For this review, take the finished solid that the model builds, in its own axes (mm). A direction names the side the tool comes from. Give positions to 0.01 mm unless a question says otherwise; leave off trailing zeros. Order: outer loops, then holes, each group sorted by start corner. A loop starts at its lowest first (then second) coordinate and runs counter-clockwise, first axis right, second up. Notation, with made-up numbers: (-34, 10.5) -> (-18, 10.5) arc R34 ccw to (-18, 46.5) -> close; hole circle Ø6 at (41, 40.25). An arc over 180 degrees is marked (long way). One line per item, written item: value. Start each with the question number.
from build123d import *

# Parameters (mm, degrees)
SKETCH2_W           = 25
SKETCH2_H           = 40
BOSS_EXTRUDE3_DEPTH = 60
SKETCH13_W          = 21
SKETCH13_H          = 42
CUT_EXTRUDE5_DEPTH  = 37
SKETCH15_W          = 25
SKETCH15_H          = 7.915590507
CUT_EXTRUDE7_DEPTH  = 7.2
SKETCH16_R          = 1.5
CUT_EXTRUDE8_DEPTH  = 8
SKETCH17_W          = 25
SKETCH17_H          = 36
CUT_EXTRUDE9_DEPTH  = 7.2
SKETCH19_W          = 20
SKETCH19_H          = 29
CUT_EXTRUDE10_DEPTH = 4
SKETCH23_R          = 2
CUT_EXTRUDE12_DEPTH = 10
SKETCH24_W          = 5.82179869
SKETCH24_H          = 4.560057011
SKETCH24_W_2        = 6.048044386
CUT_EXTRUDE14_DEPTH = 1
SKETCH25_W          = 3.2
SKETCH25_H          = 3.755693487
CUT_EXTRUDE15_DEPTH = 1
SKETCH28_R          = 1.5
BOSS_EXTRUDE4_DEPTH = 4
SKETCH29_R          = 1
CUT_EXTRUDE16_DEPTH = 10


with BuildPart() as part:
    # Sketch2 → Boss-Extrude3 (new body)
    with BuildSketch(Plane(origin=(0, 0, 0), x_dir=(1, 0, 0), z_dir=(0, 1, 0))):
        Rectangle(SKETCH2_W, SKETCH2_H)
    extrude(amount=BOSS_EXTRUDE3_DEPTH)

    # Sketch13 → Cut-Extrude5 (cut)
    with BuildSketch(Plane.XY.offset(20)):
        with Locations((-0.5, 29)):
            Rectangle(SKETCH13_W, SKETCH13_H)
    extrude(amount=-CUT_EXTRUDE5_DEPTH, mode=Mode.SUBTRACT)

    # Sketch15 → Cut-Extrude7 (cut)
    with BuildSketch(Plane.XZ):
        with Locations((0, 12.042204747)):
            Rectangle(SKETCH15_W, SKETCH15_H)
    extrude(amount=-CUT_EXTRUDE7_DEPTH, mode=Mode.SUBTRACT)

    # Sketch16 → Cut-Extrude8 (cut)
    with BuildSketch(Plane.XZ):
        with Locations(Location((0, -11.240217596, 0), (0, 0, 270))):
            Circle(SKETCH16_R)
    extrude(amount=-CUT_EXTRUDE8_DEPTH, mode=Mode.SUBTRACT)

    # Sketch17 → Cut-Extrude9 (cut)
    with BuildSketch(Plane(origin=(0, 60, 0), x_dir=(1, 0, 0), z_dir=(0, 1, 0))):
        with Locations((0, 2)):
            Rectangle(SKETCH17_W, SKETCH17_H)
    extrude(amount=-CUT_EXTRUDE9_DEPTH, mode=Mode.SUBTRACT)

    # Sketch19 → Cut-Extrude10 (cut)
    with BuildSketch(Plane(origin=(0, 52.8, 0), x_dir=(1, 0, 0), z_dir=(0, 1, 0))):
        with Locations((0, 2.255693487)):
            Rectangle(SKETCH19_W, SKETCH19_H)
    extrude(amount=-CUT_EXTRUDE10_DEPTH, mode=Mode.SUBTRACT)

    # Sketch23 → Cut-Extrude12 (cut)
    with BuildSketch(Plane.XY.offset(20)):
        with Locations((-5.5, 54)):
            Circle(SKETCH23_R)
        with Locations((4.5, 54)):
            Circle(SKETCH23_R)
        with Locations((-5.5, 4)):
            Circle(SKETCH23_R)
        with Locations((4.5, 4)):
            Circle(SKETCH23_R)
    extrude(amount=-CUT_EXTRUDE12_DEPTH, mode=Mode.SUBTRACT)

    # Sketch24 → Cut-Extrude14 (cut)
    with BuildSketch(Plane.XZ.offset(-7.2)):
        with Locations((-5.147829388, 13.719971495)):
            Rectangle(SKETCH24_W, SKETCH24_H)
        with Locations((4.519232113, 13.719971495)):
            Rectangle(SKETCH24_W_2, SKETCH24_H)
    extrude(amount=-CUT_EXTRUDE14_DEPTH, mode=Mode.SUBTRACT)

    # Sketch25 → Cut-Extrude15 (cut)
    with BuildSketch(Plane(origin=(0, 52.8, 0), x_dir=(1, 0, 0), z_dir=(0, 1, 0))):
        with Locations((-5.5, -14.122153257)):
            Rectangle(SKETCH25_W, SKETCH25_H)
        with Locations((4.5, -14.122153257)):
            Rectangle(SKETCH25_W, SKETCH25_H)
    extrude(amount=-CUT_EXTRUDE15_DEPTH, mode=Mode.SUBTRACT)

    # Sketch28 → Boss-Extrude4 (add)
    with BuildSketch(Plane(origin=(0, 0, -20), x_dir=(-1, 0, 0), z_dir=(0, 0, -1))):
        with Locations(Location((0, 40, 0), (0, 0, 180))):
            Circle(SKETCH28_R)
    extrude(amount=BOSS_EXTRUDE4_DEPTH)

    # Sketch29 → Cut-Extrude16 (cut)
    with BuildSketch(Plane.XZ):
        with Locations(Location((0, -4.240217596, 0), (0, 0, 270))):
            Circle(SKETCH29_R)
        with Locations(Location((-7, -11.240217596, 0), (0, 0, 270))):
            Circle(SKETCH29_R)
        with Locations(Location((7, -11.240217596, 0), (0, 0, 270))):
            Circle(SKETCH29_R)
    extrude(amount=-CUT_EXTRUDE16_DEPTH, mode=Mode.SUBTRACT)


solid = part.part
Q1. For pin 1 Ø0.8 at (x, y) = (4.5, 52) entering from -Z; pin 2 Ø2.5 at (x, y) = (4.5, 54) entering from +Z; pin 3 Ø8 at (x, z) = (-10, 5) entering from +Y; pin 4 Ø4 at (x, z) = (0, -11.24) entering from -Y, all flat-tipped, find the tip position at first contact; note any pin that passes through.
Q2. For line 1 along Y through (x, z) = (4.5, 17.25); line 2 along X through (y, z) = (54, 18); line 3 along X through (y, z) = (40.5, 0), list the stretches that pass through material, from the lowest coordinate up.
Q3. Take a section at C-C (y = 4). State the section outline as (x, z) points, and give its area (3 significant figures).
Q4. For faces 1 (the flat face through (0, 56, 16)), 2 (the flat face through (0, 51, 12.244)), 3 (the flat face through (-1, 50, 14)), list the 3-axis set-ups (+Z, -Z, +X, -X, +Y, -Y) from which the entire face can be reached by the end or side of a thin tool; tool diameter is ignored.
Q5. Mouldability with a two-part tool opening along Y and no side actions: class faces 4 (the flat face through (-11.3, 29.6, 20)), 5 (the flat face through (-1, 29, -17)), 6 (the flat face through (-6, 51.8, 14)), 7 (the cylindrical face through (-0.325, 41.464, -21.972)) as pulls with the +Y half, pulls with the -Y half, needs draft (parallel to the pull), parting line crosses it, or undercut.
Q6. Take a section at B-B (x = 4.5). State the section outline as (y, z) points.
Q7. Take a section at D-D (x = 0). State how many separate pieces and enclosed holes the cut face has, and give its area (3 significant figures).
Q8. Take a section at A-A (y = 54). State the section outline as (x, z) points, and give its area (3 significant figures).
Answers below:
1. pin 1: stops at z = -20
1. pin 2: stops at z = -16.76
1. pin 3: stops at y = 52.8
1. pin 4: stops at y = 0
2. line 1: y = 0 to 2, 6 to 8, 50 to 52, 56 to 60
2. line 2: x = -12.5 to -7.5, -3.5 to 2.5, 6.5 to 12.5
2. line 3: x = -12.5 to -11, 10 to 12.5
3. outline: (-12.5, -20) -> (12.5, -20) -> (12.5, 8.08) -> (-12.5, 8.08) -> close; (-12.5, 16) -> (-7.5, 16) -> (-7.5, 20) -> (-12.5, 20) -> close; (-3.5, 16) -> (2.5, 16) -> (2.5, 20) -> (-3.5, 20) -> close; (6.5, 16) -> (12.5, 16) -> (12.5, 20) -> (6.5, 20) -> close; hole circle Ø2 at (-7, -11.24); hole circle Ø3 at (0, -11.24); hole circle Ø2 at (0, -4.24); hole circle Ø2 at (7, -11.24)
3. area: 754 mm²
4. face 1: -Z, +X, -X, +Y
4. face 2: +Y
4. face 3: +Z
5. face 4: needs draft
5. face 5: undercut
5. face 6: pulls with the +Y half
5. face 7: parting line crosses it
6. outline: (0, -20) -> (52.8, -20) -> (52.8, -16.76) -> (50, -16.76) -> (50, -17) -> (8, -17) -> (8, 11.44) -> (7.2, 11.44) -> (7.2, 8.08) -> (0, 8.08) -> close; (0, 16) -> (2, 16) -> (2, 20) -> (0, 20) -> close; (6, 16) -> (8, 16) -> (8, 20) -> (6, 20) -> close; (50, 12.24) -> (51.8, 12.24) -> (51.8, 16) -> (52, 16) -> (52, 20) -> (50, 20) -> close; (56, 16) -> (60, 16) -> (60, 20) -> (56, 20) -> close
7. separate pieces: 4
7. enclosed holes: 0
7. area: 421 mm²
8. outline: (-12.5, 16) -> (-7.5, 16) -> (-7.5, 20) -> (-12.5, 20) -> close; (-3.5, 16) -> (2.5, 16) -> (2.5, 20) -> (-3.5, 20) -> close; (6.5, 16) -> (12.5, 16) -> (12.5, 20) -> (6.5, 20) -> close
8. area: 68.0 mm²
